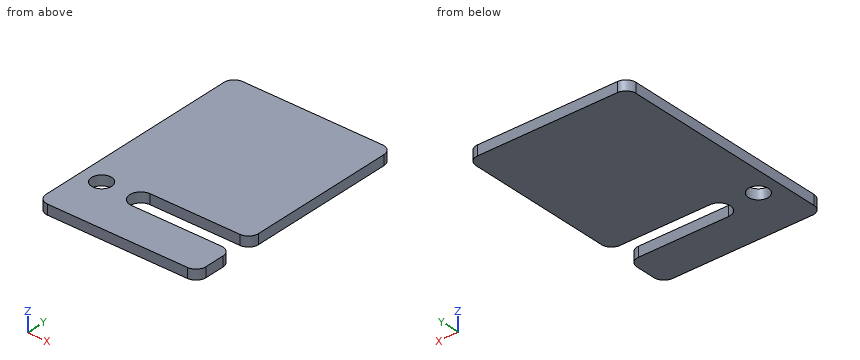
from build123d import *

# Parameters (mm, degrees)
BOSS_EXTRU_1_DEPTH      = 5
ESQUISSE3_R             = 5
ENL_V_MAT_EXTRU_1_DEPTH = 10


with BuildPart() as part:
    # Esquisse1 → Boss.-Extru.1 (new body)
    with BuildSketch(Plane.XY):
        with BuildLine():
            Line((80, 110), (80, 36))
            ThreePointArc((80, 36), (78.535533906, 32.464466094), (75, 31))
            Line((75, 31), (30, 31))
            ThreePointArc((30, 31), (24.5, 25.5), (30, 20))
            Line((30, 20), (75, 20))
            ThreePointArc((75, 20), (78.535533906, 18.535533906), (80, 15))
            Line((80, 15), (80, 5))
            ThreePointArc((80, 5), (78.535533906, 1.464466094), (75, 0))
            Line((75, 0), (5, 0))
            ThreePointArc((5, 0), (1.464466094, 1.464466094), (0, 5))
            Line((0, 5), (0, 110))
            ThreePointArc((0, 110), (1.464466094, 113.535533906), (5, 115))
            Line((5, 115), (75, 115))
            ThreePointArc((75, 115), (78.535533906, 113.535533906), (80, 110))
        make_face()
    extrude(amount=BOSS_EXTRU_1_DEPTH)

    # Esquisse3 → Enlèv. mat.-Extru.1 (cut)
    with BuildSketch(Plane(origin=(0, 0, 0), x_dir=(-1, 0, 0), z_dir=(0, 0, -1))):
        with Locations((-10.415827114, 25.5)):
            Circle(ESQUISSE3_R)
    extrude(amount=-ENL_V_MAT_EXTRU_1_DEPTH, mode=Mode.SUBTRACT)


solid = part.part
Could you check a few things on this model? Use its own coordinates, in mm. Give positions to 0.01 mm unless a question says otherwise; leave off trailing zeros. Order: outer loops, then holes, each group sorted by start corner. A loop starts at its lowest first (then second) coordinate and runs counter-clockwise, first axis right, second up.
1. Will this pin go through, and if not, where does the flat tip stop? P1, Ø3, axis at x = 54, y = 48, coming from the -Z side.
2. I need wall thicknesses on L1, parallel to Y at x = 49.5, z = 3.7; L2, parallel to Y at x = 14, z = 0.8; L3, parallel to X at y = 16, z = 3.95. Which ranges of each line are inside material? Lowest first, please.
3. Suppose I cut it at B-B (y = 25.5). List the corners of the cut face in (x, z) for me, plus the area to 3 significant figures.
4. Suppose I cut it at C-C (z = 3.8). List the corners of the cut face in (x, y) for me, plus the area to 3 significant figures.
5. Suppose I cut it at A-A (x = 43). List the corners of the cut face in (y, z) for me, plus the area to 3 significant figures.
Solved:
1. P1: stops at z = 0
2. L1: y = 0 to 20, 31 to 115
2. L2: y = 0 to 22.01, 28.99 to 115
2. L3: x = 0 to 79.9
3. outline: (0, 0) - (5.42, 0) - (5.42, 5) - (0, 5) - close; (15.42, 0) - (24.5, 0) - (24.5, 5) - (15.42, 5) - close
3. area: 72.5 mm2
4. outline: (0, 5) arc R5 ccw to (5, 0) - (75, 0) arc R5 ccw to (80, 5) - (80, 15) arc R5 ccw to (75, 20) - (30, 20) arc R5.5 cw to (30, 31) - (75, 31) arc R5 ccw to (80, 36) - (80, 110) arc R5 ccw to (75, 115) - (5, 115) arc R5 ccw to (0, 110) - close; hole circle Ø10 at (10.42, 25.5)
4. area: 8,490 mm2
5. outline: (0, 0) - (20, 0) - (20, 5) - (0, 5) - close; (31, 0) - (115, 0) - (115, 5) - (31, 5) - close
5. area: 520 mm2
